Study the drawing (mm; zero at the part's minimum x, y, z) and answer. A direction names the side the tool comes from. Give positions to 0.01 mm unless a question says otherwise; leave off trailing zeros. Order: outer loops, then holes, each group sorted by start corner. A loop starts at its lowest first (then second) coordinate and runs counter-clockwise, first axis right, second up.
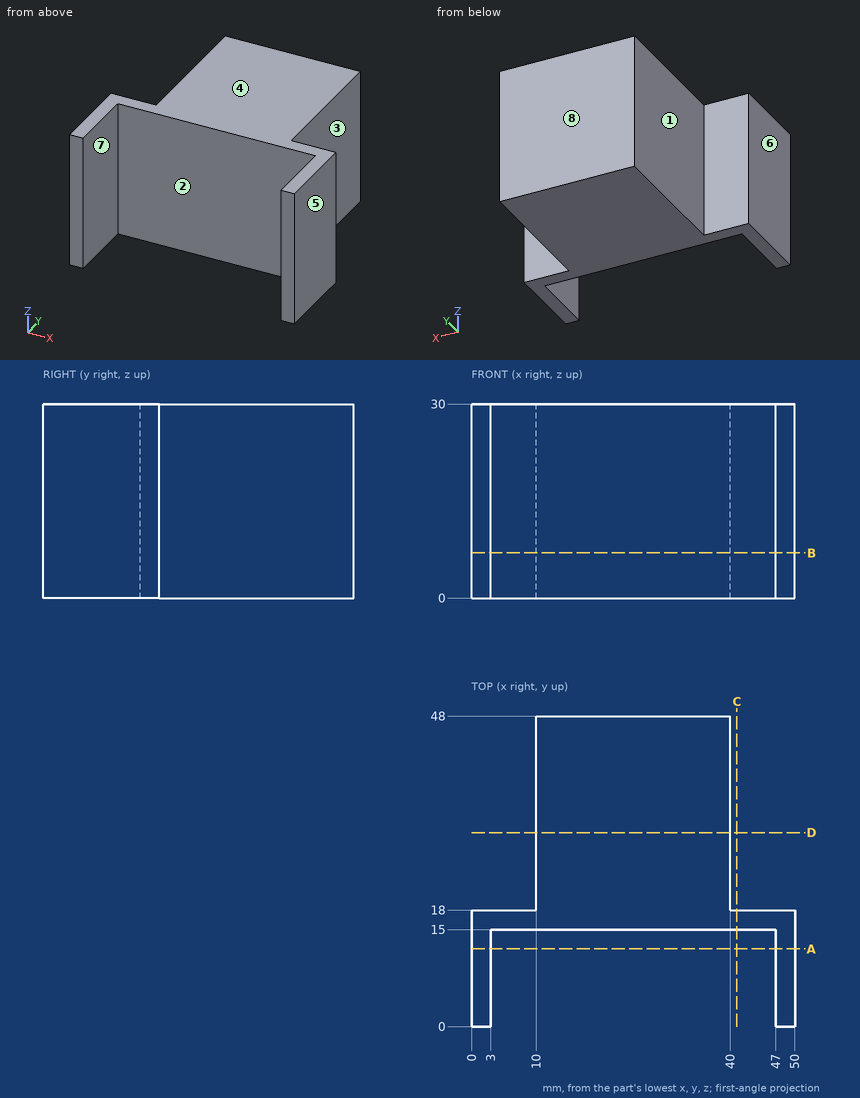
1) Find section C-C (x = 41). Write down the section's boundary in (y, z), then the cut area to 3 significant figures.
Geometry says:
outline: (15, 0) - (18, 0) - (18, 30) - (15, 30) - close
area: 90.0 mm2
2) A tool of negligible diameter and unlimited length cuts with its end or side. For the marked faces 1, 2, 3 and 4, from which of +Z, -Z, +X, -X, +Y, -Y can it reach the whole face along a straight path? Write none if from no direction.
Geometry says:
face 1: +Z, -Z, -X, +Y
face 2: +Z, -Z, -Y
face 3: +Z, -Z, +X, +Y
face 4: +Z, +X, -X, +Y, -Y
3) Straight lines are drawn through the part: probe 1 along X at (y, z) = (3, 11); probe 2 along Y at (x, z) = (28, 27); probe 3 along X at (y, z) = (41.5, 24.75). For each, find the intervals that lie inside material, in ascending order.
Geometry says:
probe 1: x = 0 to 3, 47 to 50
probe 2: y = 15 to 48
probe 3: x = 10 to 40
4) Find section D-D (y = 30). Write down the section's boundary in (x, z).
Geometry says:
outline: (10, 0) - (40, 0) - (40, 30) - (10, 30) - close
5) Find section A-A (y = 12). Write down the section's boundary in (x, z).
Geometry says:
outline: (0, 0) - (3, 0) - (3, 30) - (0, 30) - close; (47, 0) - (50, 0) - (50, 30) - (47, 30) - close
6) Given P1, Ø1.5, axis at x = 43, z = 22.5, coming from the +Y side; P2, Ø15, axis at y = 37.5, z = 10.5, coming from the +X side; P3, Ø6, axis at x = 12.5, z = 11, coming from the -Y side, each flat-ended and moving along its own axis, determine where each tip first touches the part or whether it passes through.
Geometry says:
P1: stops at y = 18
P2: stops at x = 40
P3: stops at y = 15
7) Find section B-B (z = 7). Write down the section's boundary in (x, y).
Geometry says:
outline: (0, 0) - (3, 0) - (3, 15) - (47, 15) - (47, 0) - (50, 0) - (50, 18) - (40, 18) - (40, 48) - (10, 48) - (10, 18) - (0, 18) - close
8) For a pull along X with two mould halves and no side action, classify the marked faces 5, 6, 7 and 8 as +X half, -X half, draft (parallel to the pull), parting line (faces both ways), or undercut.
Geometry says:
face 5: +X half
face 6: -X half
face 7: undercut
face 8: draft
